Here's how the part is built. I have some questions about the finished solid (model axes, mm). A direction names the side the tool comes from. Coordinates: 2 decimals unless noted, no trailing zeros. Write each loop counter-clockwise with the first axis right and the second up, starting at its lowest first coordinate (ties: lowest second). Pieces come first, ordered by that corner, then holes. Notation, with made-up numbers: (74.5, 27) -> (88.5, 27) arc R5 cw to (88.5, 35) -> close; hole circle Ø4 at (64, 62). An arc over 180 degrees is marked (long way). Use CSV: the item, a comma, the result in double quotes. Start each with the question number.
```python
from build123d import *

# Parameters (mm, degrees)
F0_W          = 38.661484
F0_H          = 119.03402
F1_DEPTH      = 12.7
F3_R          = 12.7
F4_DEPTH      = 183.44656
F4_DEPTH_BACK = 8.28374
F2_R          = 9.525
F5_DEPTH      = 94.33232
F6_W          = 221.033588
F6_H          = 240.64786
F7_DEPTH      = 25.4
F8_W          = 220.933356
F8_H          = 245.975703
F9_DEPTH      = 25.4


with BuildPart() as f1:
    # F0 (on Front) → F1 (new body)
    with BuildSketch(Plane.XZ):
        Rectangle(F0_W, F0_H)
    extrude(amount=F1_DEPTH)

    # F3 (on Front) → F4 (join, two sides)
    with BuildSketch(Plane.XZ) as f4_sk:
        with Locations((0, -35.640396)):
            Circle(F3_R)
    extrude(amount=-F4_DEPTH)
    extrude(f4_sk.sketch, amount=-F4_DEPTH_BACK)

    # F2 (on Front) → F5 (join)
    with BuildSketch(Plane.XZ):
        with Locations((0, 35.779871)):
            Circle(F2_R)
    extrude(amount=F5_DEPTH)

    # F6 (on Front) → F7 (join)
    with BuildSketch(Plane.XZ):
        with Locations((5.755909, -41.401114)):
            Rectangle(F6_W, F6_H)
    extrude(amount=-F7_DEPTH)

    # F8 (on Top) → F9 (join)
    with BuildSketch(Plane.XY):
        with Locations((5.063448, 122.987851)):
            Rectangle(F8_W, F8_H)
    extrude(amount=F9_DEPTH)


solid = f1.part
```
Item 1: If I drill on line 1 along Y through (x, z) = (-84, -91); line 2 along X through (y, z) = (-6, 25.5), over which ranges is the centre line in solid material (lowest first)?
Item 2: I want a section at D-D on y = 195. Please give me the cut outline in (x, z), then the cut area to 3 significant figures.
Item 3: I want a section at B-B on x = 94. Please give me the cut outline in (y, z), then the cut area to 3 significant figures.
Item 4: I want a section at C-C on y = 133. Please give me the cut outline in (x, z), then the cut area to 3 significant figures.
Item 5: I want a section at A-A on z = -6.5. Please give me the cut outline in (x, y).
Item 6: Which directions (+Z, -Z, +X, -X, +Y, -Y) give clear straight access to the entire face, cutting with the end or side of a thin tool? Please do faces 1 (the flat face through (19.331, -6, -1)), 2 (the flat face through (-63, 0, 13)), 3 (the cylindrical face through (-1.65, 103.32, -23.05)), 4 (the flat face through (0, 183.447, -35)), 5 (the flat face through (-104.761, 13, -82)).
Item 7: I'm going to push flat-ended pins straight in: pin 1 (10 mm diameter, centred on x = 1, y = -3.5, fed in from -Z); pin 2 (20.5 mm diameter, centred on y = 162.5, z = 13, fed in from +X); pin 3 (20.5 mm diameter, centred on x = 1.5, z = -41, fed in from +Y); pin 4 (6.5 mm diameter, centred on y = -7, z = -2.5, fed in from +X). Where does each tip first touch, or does it pass through?
Geometry says:
1,line 1,"0 to 25.4"
1,line 2,"-19.33 to 19.33"
2,outline,"(-105.4, 0) -> (115.53, 0) -> (115.53, 25.4) -> (-105.4, 25.4) -> close"
2,area,"5,610 mm2"
3,outline,"(0, -161.73) -> (25.4, -161.73) -> (25.4, 0) -> (245.98, 0) -> (245.98, 25.4) -> (25.4, 25.4) -> (25.4, 78.92) -> (0, 78.92) -> close"
3,area,"11,700 mm2"
4,outline,"(-105.4, 0) -> (115.53, 0) -> (115.53, 25.4) -> (-105.4, 25.4) -> close; circle Ø25.4 at (0, -35.64)"
4,area,"6,120 mm2"
5,outline,"(-104.76, 0) -> (-19.33, 0) -> (-19.33, -12.7) -> (19.33, -12.7) -> (19.33, 0) -> (116.27, 0) -> (116.27, 25.4) -> (-104.76, 25.4) -> close"
6,face 1,"+Z, -Z, +X, -Y"
6,face 2,"+Z, -Z, -X, -Y"
6,face 3,"+Y"
6,face 4,"-Z, +X, -X, +Y"
6,face 5,"-Z, -X, +Y, -Y"
7,pin 1,"z = -161.73"
7,pin 2,"x = 115.53"
7,pin 3,"y = 183.45"
7,pin 4,"x = 19.33"
